```python
from build123d import *

# Parameters (mm, degrees)
ESQUISSE2_R             = 159
ESQUISSE2_R_2           = 151
BOSS_EXTRU_1_DEPTH      = 55
ESQUISSE3_R             = 155
ENL_V_MAT_EXTRU_1_DEPTH = 4


with BuildPart() as part:
    # Esquisse2 → Boss.-Extru.1 (new body, symmetric)
    with BuildSketch(Plane(origin=(0, 0, 0), x_dir=(1, 0, 0), z_dir=(0, 1, 0))):
        Circle(ESQUISSE2_R)
        Circle(ESQUISSE2_R_2, mode=Mode.SUBTRACT)
    extrude(amount=BOSS_EXTRU_1_DEPTH, both=True)

    # Esquisse3 → Enlèv. mat.-Extru.1 (cut)
    with BuildSketch(Plane(origin=(0, 55, 0), x_dir=(1, 0, 0), z_dir=(0, 1, 0))):
        Circle(ESQUISSE3_R)
    enl_v_mat_extru_1 = extrude(amount=-ENL_V_MAT_EXTRU_1_DEPTH, mode=Mode.SUBTRACT)

    # Symétrie1: Enlèv. mat.-Extru.1 across plane
    add(enl_v_mat_extru_1.mirror(Plane.ZX), mode=Mode.SUBTRACT)


solid = part.part
```
The listing builds one solid part. Answer for the finished solid, in the listing's coordinates (mm). A direction names the side the tool comes from. Round coordinates to 2 decimals unless told otherwise and drop trailing zeros. Write each loop counter-clockwise with the first axis right and the second up, starting at its lowest first coordinate (ties: lowest second). Pieces come first, ordered by that corner, then holes. Notation, with made-up numbers: (1, 59) -> (6, 59) arc R26 ccw to (6, 96) -> close; hole circle Ø4 at (19.25, -14). An arc over 180 degrees is marked (long way). Use CSV: the item, a comma, the result in double quotes. Start each with the question number.
(1) Section C-C on y = -5 is taken. Give the vertices of the cut face in (x, z), then the cut area to 3 significant figures.
(2) Which of the six approach directions +Z, -Z, +X, -X, +Y, -Y give full straight-line access (tool end or side, diameter ignored) to faces 1 (the face through (-33.601, -53.028, 151.314)), 2 (the face through (35, -55, 152)), 3 (the face through (34, 51, 149))?
(3) Consider L1, parallel to Z at x = 0, y = -7; L2, parallel to Z at x = 0, y = 52. Determine where each line is inside the solid, lowest interval first. Write a range as from..to.
(4) The mould has two halves that part along Z. Classify faces 4 (the face through (-20.699, 0.77, -157.647)), 5 (the face through (35, 55, 152)), 6 (the face through (-33.601, 53.028, 151.314)): released by +Z, released by -Z, zero draft, split by the parting line, or undercut.
(5) Each of these flat-tipped pins is pushed along its axis until it touches: pin 1 (10 mm diameter, centred on y = -10.5, z = -126, fed in from -X); pin 2 (1.5 mm diameter, centred on x = -71.5, y = -14.5, fed in from -Z); pin 3 (3 mm diameter, centred on y = 17, z = 102, fed in from +X). Where does it stop, or does it pass through?
(6) Section A-A on z = 9 is taken. Give the vertices of the cut face in (x, y), then the cut area to 3 significant figures.
(7) Section B-B on x = 0 is taken. Give the vertices of the cut face in (y, z), then the cut area to 3 significant figures.
A:
1,outline,"circle Ø318 at (0, 0); hole circle Ø302 at (0, 0)"
1,area,"7,790 mm²"
2,face 1,"-Y"
2,face 2,"+Z, -Z, +X, -X, -Y"
2,face 3,"+Y"
3,L1,"z = -159..-151, 151..159"
3,L2,"z = -159..-155, 155..159"
4,face 4,"split by the parting line"
4,face 5,"zero draft"
4,face 6,"undercut"
5,pin 1,"stops at x = -103.15"
5,pin 2,"stops at z = -142.39"
5,pin 3,"stops at x = 123.21"
6,outline,"(-158.75, -55) -> (-154.74, -55) -> (-154.74, -51) -> (-150.73, -51) -> (-150.73, 51) -> (-154.74, 51) -> (-154.74, 55) -> (-158.75, 55) -> close; (150.73, -51) -> (154.74, -51) -> (154.74, -55) -> (158.75, -55) -> (158.75, 55) -> (154.74, 55) -> (154.74, 51) -> (150.73, 51) -> close"
6,area,"1,700 mm²"
7,outline,"(-55, -159) -> (55, -159) -> (55, -155) -> (51, -155) -> (51, -151) -> (-51, -151) -> (-51, -155) -> (-55, -155) -> close; (-55, 155) -> (-51, 155) -> (-51, 151) -> (51, 151) -> (51, 155) -> (55, 155) -> (55, 159) -> (-55, 159) -> close"
7,area,"1,700 mm²"
